from build123d import *

# Parameters (mm, degrees)
CROQUIS1_W                          = 62.738
CROQUIS1_H                          = 482.6
CROQUIS1_R                          = 3.9624
BRIDA_BASE1_DEPTH                   = 1.524
BRIDA_DE_ARISTA1_STRIP_W            = 9.144
BRIDA_DE_ARISTA1_STRIP_H            = 1.524
BRIDA_DE_ARISTA1_STRIP_CUT_DEPTH    = 438.15
BRIDA_DE_ARISTA1_RELIEF_W           = 9.2964
BRIDA_DE_ARISTA1_RELIEF_H           = 0.1524
BRIDA_DE_ARISTA1_RELIEF_CUT_DEPTH   = 1.524
BRIDA_DE_ARISTA1_STRIP_2_W          = 9.144
BRIDA_DE_ARISTA1_STRIP_2_H          = 1.524
BRIDA_DE_ARISTA1_STRIP_CUT_2_DEPTH  = 438.15
BRIDA_DE_ARISTA1_RELIEF_2_W         = 9.2964
BRIDA_DE_ARISTA1_RELIEF_2_H         = 0.1524
BRIDA_DE_ARISTA1_RELIEF_CUT_2_DEPTH = 1.524
BRIDA_DE_ARISTA1_DEPTH              = 438.15
BRIDA_DE_ARISTA1_BEND_DEPTH         = 438.15
CROQUIS15_R                         = 3.9624
CORTAR_EXTRUIR1_DEPTH               = 244.760777495


# Sheet-metal steps are written as plain solids
with BuildPart() as part:
    # Croquis1 → Brida base1 (new body)
    with BuildSketch(Plane.XY):
        Rectangle(CROQUIS1_W, CROQUIS1_H)
        with Locations((0.381, 231.775)):
            Circle(CROQUIS1_R, mode=Mode.SUBTRACT)
        with Locations((-0.381, -231.775)):
            Circle(CROQUIS1_R, mode=Mode.SUBTRACT)
    extrude(amount=-BRIDA_BASE1_DEPTH)

    # Brida de arista1 strip (across the edge) → Brida de arista1 strip cut (cut)
    with BuildSketch(Plane(origin=(31.369, -219.075, 0), x_dir=(-1, 0, 0), z_dir=(0, 1, 0))):
        with Locations((-1.524, -0.762)):
            Rectangle(BRIDA_DE_ARISTA1_STRIP_W, BRIDA_DE_ARISTA1_STRIP_H)
    extrude(amount=BRIDA_DE_ARISTA1_STRIP_CUT_DEPTH, mode=Mode.SUBTRACT)

    # Brida de arista1 relief (on the sheet) → Brida de arista1 relief cut (cut)
    with BuildSketch(Plane(origin=(28.321, -219.075, 0), x_dir=(-1, 0, 0), z_dir=(0, 0, 1))):
        with Locations((-4.4958, 0.0762)):
            Rectangle(BRIDA_DE_ARISTA1_RELIEF_W, BRIDA_DE_ARISTA1_RELIEF_H)
        with Locations((-4.4958, -438.2262)):
            Rectangle(BRIDA_DE_ARISTA1_RELIEF_W, BRIDA_DE_ARISTA1_RELIEF_H)
    extrude(amount=-BRIDA_DE_ARISTA1_RELIEF_CUT_DEPTH, mode=Mode.SUBTRACT)

    # Brida de arista1 strip 2 (across the edge) → Brida de arista1 strip cut 2 (cut)
    with BuildSketch(Plane(origin=(-31.369, 219.075, 0), x_dir=(1, 0, 0), z_dir=(0, -1, 0))):
        with Locations((-1.524, -0.762)):
            Rectangle(BRIDA_DE_ARISTA1_STRIP_2_W, BRIDA_DE_ARISTA1_STRIP_2_H)
    extrude(amount=BRIDA_DE_ARISTA1_STRIP_CUT_2_DEPTH, mode=Mode.SUBTRACT)

    # Brida de arista1 relief 2 (on the sheet) → Brida de arista1 relief cut 2 (cut)
    with BuildSketch(Plane(origin=(-28.321, 219.075, 0), x_dir=(1, 0, 0), z_dir=(0, 0, 1))):
        with Locations((-4.4958, 0.0762)):
            Rectangle(BRIDA_DE_ARISTA1_RELIEF_2_W, BRIDA_DE_ARISTA1_RELIEF_2_H)
        with Locations((-4.4958, -438.2262)):
            Rectangle(BRIDA_DE_ARISTA1_RELIEF_2_W, BRIDA_DE_ARISTA1_RELIEF_2_H)
    extrude(amount=-BRIDA_DE_ARISTA1_RELIEF_CUT_2_DEPTH, mode=Mode.SUBTRACT)

    # Brida de arista1 section (across the edge) → Brida de arista1 (add)
    with BuildSketch(Plane(origin=(31.369, -219.075, 0), x_dir=(-1, 0, 0), z_dir=(0, 1, 0))):
        with BuildLine():
            Line((0, 1.524), (0, 14.478))
            Line((0, 14.478), (1.524, 14.478))
            Line((1.524, 14.478), (1.524, 1.524))
            ThreePointArc((1.524, 1.524), (1.970369265, 0.446369265), (3.048, 0))
            Line((3.048, 0), (3.048, -1.524))
            ThreePointArc((3.048, -1.524), (0.892738531, -0.631261469), (0, 1.524))
        make_face()
    extrude(amount=BRIDA_DE_ARISTA1_DEPTH)

    # Brida de arista1 section 2 (across the edge) → Brida de arista1 bend (add)
    with BuildSketch(Plane(origin=(-31.369, 219.075, 0), x_dir=(1, 0, 0), z_dir=(0, -1, 0))):
        with BuildLine():
            Line((0, 1.524), (0, 14.478))
            Line((0, 14.478), (1.524, 14.478))
            Line((1.524, 14.478), (1.524, 1.524))
            ThreePointArc((1.524, 1.524), (1.970369265, 0.446369265), (3.048, 0))
            Line((3.048, 0), (3.048, -1.524))
            ThreePointArc((3.048, -1.524), (0.892738531, -0.631261469), (0, 1.524))
        make_face()
    extrude(amount=BRIDA_DE_ARISTA1_BEND_DEPTH)

    # Croquis15 → Cortar-Extruir1 (cut, through all)
    with BuildSketch(Plane.XY):
        with Locations((-31.7754, 231.775)):
            Circle(CROQUIS15_R)
        with Locations((-31.7754, -231.775)):
            Circle(CROQUIS15_R)
        with Locations((31.7754, -231.775)):
            Circle(CROQUIS15_R)
        with Locations((31.7754, 231.775)):
            Circle(CROQUIS15_R)
    extrude(amount=-CORTAR_EXTRUIR1_DEPTH, mode=Mode.SUBTRACT)


solid = part.part
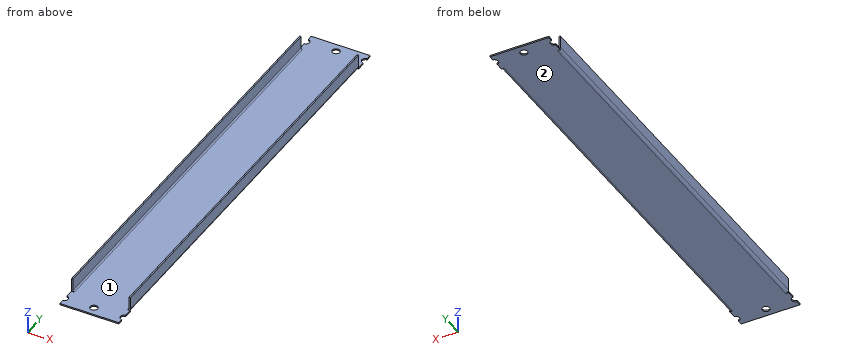
Design review of the part built by this model. Coordinates are the model's own, in mm. Face numbers are marked on the shaded views. Round coordinates to 2 decimals unless told otherwise and drop trailing zeros. Write each loop counter-clockwise with the first axis right and the second up, starting at its lowest first coordinate (ties: lowest second). Pieces come first, ordered by that corner, then holes.
Item 1: Consider section B-B on y = 148.5. Give the boundary of the cut face in (x, z) (3 decimals).
Item 2: Consider section C-C on x = -18. Give the boundary of the cut face in (y, z), and give its area (3 significant figures).
Item 3: For pin 1 Ø2.5 at (x, z) = (30.5, 9) entering from -Y (3 decimals); pin 2 Ø10.5 at (x, y) = (-0.381, -231.775) entering from -Z; pin 3 Ø2 at (x, y) = (-14, 122) entering from +Z; pin 4 Ø3.5 at (x, z) = (-29.5, 6) entering from +Y (3 decimals), all flat-tipped, find the tip position at first contact; note any pin that passes through.
Item 4: Consider section A-A on z = 11.5. Give the boundary of the cut face in (x, y) (3 decimals), and give its area (3 significant figures).
Item 5: Draft analysis for pull direction X (two halves, no side actions). For the marked faces 1 and 2, state which applies: released by +X, released by -X, zero draft, split by the parting line, or undercut.
Item 6: Wall thickness on L1, parallel to X at y = 120.5, z = 4.75 (3 decimals); L2, parallel to Z at x = -3, y = 128; L3, parallel to X at y = 211.5, z = 0.75: over which ranges is each line inside the solid? List them lowest first.
Check values:
1. outline: (-31.369, 1.524) arc R3.048 ccw to (-28.321, -1.524) - (28.321, -1.524) arc R3.048 ccw to (31.369, 1.524) - (31.369, 14.478) - (29.845, 14.478) - (29.845, 1.524) arc R1.524 cw to (28.321, 0) - (-28.321, 0) arc R1.524 cw to (-29.845, 1.524) - (-29.845, 14.478) - (-31.369, 14.478) - close
2. outline: (-241.3, -1.52) - (241.3, -1.52) - (241.3, 0) - (-241.3, 0) - close
2. area: 735 mm2
3. pin 1: stops at y = -219.075
3. pin 2: stops at z = -1.52
3. pin 3: stops at z = 0
3. pin 4: stops at y = 219.075
4. outline: (-31.369, -219.075) - (-29.845, -219.075) - (-29.845, 219.075) - (-31.369, 219.075) - close; (29.845, -219.075) - (31.369, -219.075) - (31.369, 219.075) - (29.845, 219.075) - close
4. area: 1,340 mm2
5. face 1: undercut
5. face 2: zero draft
6. L1: x = -31.369 to -29.845, 29.845 to 31.369
6. L2: z = -1.52 to 0
6. L3: x = -31.27 to -29.63, 29.63 to 31.27
